Here's how the part is built. I have some questions about the finished solid (model axes, mm). Face numbers are marked on the shaded views. A direction names the side the tool comes from. Coordinates: 2 decimals unless noted, no trailing zeros. Write each loop counter-clockwise with the first axis right and the second up, starting at its lowest first coordinate (ties: lowest second). Pieces come first, ordered by that corner, then holes. Notation, with made-up numbers: (29, -1) -> (45, -1) arc R19 cw to (45, 16) -> close; hole circle Ø6 at (82.25, 82). An arc over 180 degrees is marked (long way). Use a Markdown table: item, result. Add a question column.
```python
from build123d import *

# Parameters (mm, degrees)
SKETCH1_W                  = 36.2966
SKETCH1_H                  = 80.2132
BOSS_BASE_DEPTH            = 2.1717
SKETCH3_W                  = 36.2966
SKETCH3_H                  = 2.1717
BOSS_LIP_DEPTH             = 23.25116
F_4_0_209_DIAMETER_HOLE1_D = 5.3086
F_4_0_209_DIAMETER_HOLE2_D = 5.3086
SKETCH19_W                 = 3.0734
SKETCH19_H                 = 66.04
CUT_EXTRUDE1_DEPTH         = 50.784702448
FILLET1_R                  = 3.81
FILLET4_R                  = 0.635


with BuildPart() as part:
    # Sketch1 → Boss-Base (new body)
    with BuildSketch(Plane(origin=(0, 0, 0), x_dir=(1, 0, 0), z_dir=(0, 1, 0))):
        Rectangle(SKETCH1_W, SKETCH1_H)
    extrude(amount=BOSS_BASE_DEPTH)

    # Sketch3 → Boss-Lip (add)
    with BuildSketch(Plane(origin=(0, 2.1717, 0), x_dir=(1, 0, 0), z_dir=(0, 1, 0))):
        with Locations((0, 39.02075)):
            Rectangle(SKETCH3_W, SKETCH3_H)
    extrude(amount=BOSS_LIP_DEPTH)

    # #4 (0.209) Diameter Hole1 (through all)
    with Locations(Plane(origin=(0, 2.1717, 0), x_dir=(1, 0, 0), z_dir=(0, 1, 0))):
        with Locations((0, -29.9466), (0, 10.0584)):
            Hole(F_4_0_209_DIAMETER_HOLE1_D / 2)

    # #4 (0.209) Diameter Hole2 (through all)
    with Locations(Plane.XY.offset(-37.9349)):
        with Locations((10.2743, 17.54886), (-10.2743, 17.54886)):
            Hole(F_4_0_209_DIAMETER_HOLE2_D / 2)

    # Sketch19 → Cut-Extrude1 (cut, through all)
    with BuildSketch(Plane(origin=(0, 2.1717, 0), x_dir=(1, 0, 0), z_dir=(0, 1, 0))):
        with Locations((16.6116, -7.0866)):
            Rectangle(SKETCH19_W, SKETCH19_H)
        with Locations((-16.6116, -7.0866)):
            Rectangle(SKETCH19_W, SKETCH19_H)
    extrude(amount=-CUT_EXTRUDE1_DEPTH, mode=Mode.SUBTRACT)

    # Fillet1
    # the kernel refuses this fillet: 3.81 mm, written as the material it adds along each edge
    with BuildSketch(Plane(origin=(18.1483, 2.1717, -37.9349), x_dir=(0, 0, 1), z_dir=(-1, 0, 0))) as fillet1_piece_1:
        with BuildLine():
            CenterArc((FILLET1_R, FILLET1_R), FILLET1_R, 180, 90)
            Line((0, FILLET1_R), (0, 0))
            Line((0, 0), (FILLET1_R, 0))
        make_face()
    extrude(amount=36.2966)
    # the kernel refuses this fillet: 3.81 mm, written as the material it takes off along each edge
    with BuildSketch(Plane(origin=(-18.1483, 11.51699308, -25.9334), x_dir=(0, 0, -1), z_dir=(0, -1, 0))) as fillet1_2_piece_1:
        with BuildLine():
            CenterArc((3.738117232, 3.81), FILLET1_R, 191.147377986, 78.852622014)
            Line((0, 3.0734), (0, 0))
            Line((0, 0), (3.738117232, 0))
        make_face()
    extrude(amount=20.86228616, mode=Mode.SUBTRACT)
    with BuildSketch(Plane(origin=(18.1483, 11.51699308, -25.9334), x_dir=(-1, 0, 0), z_dir=(0, -1, 0))) as fillet1_2_piece_2:
        with BuildLine():
            CenterArc((3.81, 3.738117232), FILLET1_R, 180, 78.852622014)
            Line((0, 3.738117232), (0, 0))
            Line((0, 0), (3.0734, 0))
        make_face()
    extrude(amount=20.86228616, mode=Mode.SUBTRACT)
    with BuildSketch(Plane(origin=(15.0749, 11.6967, 40.1066), x_dir=(-1, 0, 0), z_dir=(0, -1, 0))) as fillet1_2_piece_3:
        with BuildLine():
            CenterArc((FILLET1_R, FILLET1_R), FILLET1_R, 180, 90)
            Line((0, FILLET1_R), (0, 0))
            Line((0, 0), (FILLET1_R, 0))
        make_face()
    extrude(amount=21.2217, mode=Mode.SUBTRACT)
    with BuildSketch(Plane(origin=(-15.0749, 11.6967, 40.1066), x_dir=(1, 0, 0), z_dir=(0, -1, 0)), Plane(origin=(-18.1483, 25.42286, -28.4099), x_dir=(0, -1, 0), z_dir=(0, 0, -1)), Plane(origin=(18.1483, 25.42286, -49.6316), x_dir=(0, -1, 0), z_dir=(0, 0, 1))) as fillet1_2_piece_4:
        with BuildLine():
            CenterArc((FILLET1_R, -FILLET1_R), FILLET1_R, 90, 90)
            Line((0, -FILLET1_R), (0, 0))
            Line((0, 0), (FILLET1_R, 0))
        make_face()
    extrude(amount=21.2217, mode=Mode.SUBTRACT)
    with BuildSketch(Plane(origin=(-27.6733, 0, -40.1066), x_dir=(0, 0, 1), z_dir=(1, 0, 0))) as fillet1_2_piece_5:
        with BuildLine():
            CenterArc((FILLET1_R, -FILLET1_R), FILLET1_R, 90, 90)
            Line((0, -FILLET1_R), (0, 0))
            Line((0, 0), (FILLET1_R, 0))
        make_face()
    extrude(amount=55.3466, mode=Mode.SUBTRACT)

    # Fillet4
    fillet4_edges = [part.edges().sort_by_distance(p)[0] for p in [
        (18.1483, 3.287623164, -36.818976836),
        (-18.1483, 3.287623164, -36.818976836),
        (15.0749, 0, 5.1816),
        (15.0749, 2.1717, 5.1816),
        (18.1483, 13.79728, -37.9349),
        (0, 25.42286, -37.9349),
        (-18.1483, 13.79728, -37.9349),
        (17.032376836, 24.306936836, -37.9349),
        (-17.032376836, 24.306936836, -37.9349),
        (18.1483, 2.1717, -31.898208616),
        (-18.1483, 2.1717, -31.898208616),
        (-15.0749, 2.1717, 5.1816),
        (0, 2.1717, 40.1066),
        (-17.281304077, 2.1717, -27.251842254),
        (17.281304077, 2.1717, -27.251842254),
        (13.958976836, 2.1717, 38.990676836),
        (-13.958976836, 2.1717, 38.990676836),
        (-18.1483, 12.71143, -40.1066),
        (0, 25.42286, -40.1066),
        (18.1483, 12.71143, -40.1066),
        (17.032376836, 24.306936836, -40.1066),
        (-17.032376836, 24.306936836, -40.1066),
        (-18.1483, 0, -32.984058616),
        (-18.1483, 1.115923164, -38.990676836),
        (0, 0, 40.1066),
        (-15.0749, 0, 5.1816),
        (18.1483, 0, -32.984058616),
        (-17.281304077, 0, -27.251842254),
        (17.281304077, 0, -27.251842254),
        (13.958976836, 0, 38.990676836),
        (-13.958976836, 0, 38.990676836),
        (18.1483, 1.115923164, -38.990676836),
    ]]
    fillet(fillet4_edges, radius=FILLET4_R)


solid = part.part
```
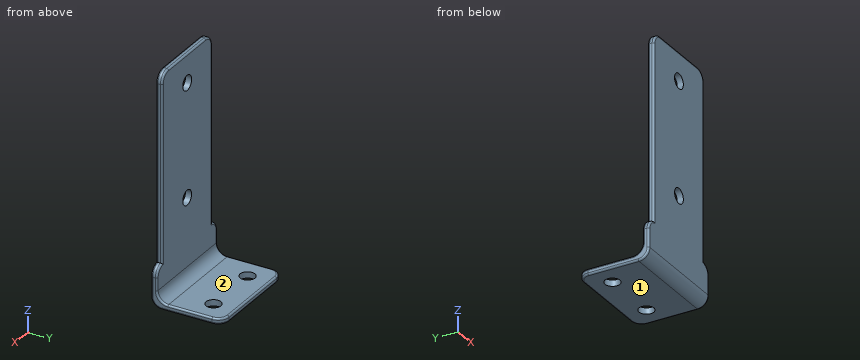
Q1. Which directions (+Z, -Z, +X, -X, +Y, -Y) give clear straight access to the entire face, cutting with the end or side of a thin tool? Please do the marked faces 1 and 2.
Q2. Suppose I cut it at D-D, the plane x = 5. Write out the boundary of the cut face in (y, z) (3 decimals).
Q3. Suppose I cut it at A-A, the plane x = 0. Write out the boundary of the cut face in (y, z) (3 decimals).
Q4. Suppose I cut it at B-B, the plane y = 16.5. Write out the boundary of the cut face in (x, z) (3 decimals).
Q5. Suppose I cut it at C-C, the plane z = 24. Write out the boundary of the cut face in (x, y) (3 decimals), and give its area (3 significant figures).
Q6. Please list where these lines run through material, in increasing order: line 1 (Z direction, x = 0, y = 1.45); line 2 (Y direction, x = 0, z = 8.5); line 3 (Z direction, x = 0, y = 1.25).
Q7. Will these pins go through, and if not, where does the flat tip stop? pin 1 (4 mm diameter, centred on x = 10.27, y = 17.55, fed in from -Z); pin 2 (3 mm diameter, centred on x = 9.5, z = -1.5, fed in from +Y); pin 3 (0.7 mm diameter, centred on y = 1, z = 10.5, fed in from +X); pin 4 (2 mm diameter, centred on x = -8, y = 19, fed in from +Z).
Answer key:
| question | item | result |
|---|---|---|
| 1 | face 1 | -Z, +X, -X, +Y, -Y |
| 1 | face 2 | +Z, +X, -X, +Y |
| 2 | outline | (0, -36.297) arc R3.81 ccw to (3.81, -40.107) -> (24.788, -40.107) arc R0.635 ccw to (25.423, -39.472) -> (25.423, -38.57) arc R0.635 ccw to (24.788, -37.935) -> (5.982, -37.935) arc R3.81 cw to (2.172, -34.125) -> (2.172, 39.472) arc R0.635 ccw to (1.537, 40.107) -> (0.635, 40.107) arc R0.635 ccw to (0, 39.472) -> close |
| 3 | outline | (0, -36.297) arc R3.81 ccw to (3.81, -40.107) -> (24.788, -40.107) arc R0.635 ccw to (25.423, -39.472) -> (25.423, -38.57) arc R0.635 ccw to (24.788, -37.935) -> (5.982, -37.935) arc R3.81 cw to (2.172, -34.125) -> (2.172, -12.713) -> (0, -12.713) -> close; (0, -7.404) -> (2.172, -7.404) -> (2.172, 27.292) -> (0, 27.292) -> close; (0, 32.601) -> (2.172, 32.601) -> (2.172, 39.472) arc R0.635 ccw to (1.537, 40.107) -> (0.635, 40.107) arc R0.635 ccw to (0, 39.472) -> close |
| 4 | outline | (-18.148, -39.472) arc R0.635 ccw to (-17.513, -40.107) -> (-12.713, -40.107) -> (-12.713, -37.935) -> (-17.513, -37.935) arc R0.635 ccw to (-18.148, -38.57) -> close; (-7.836, -40.107) -> (7.836, -40.107) -> (7.836, -37.935) -> (-7.836, -37.935) -> close; (12.713, -40.107) -> (17.513, -40.107) arc R0.635 ccw to (18.148, -39.472) -> (18.148, -38.57) arc R0.635 ccw to (17.513, -37.935) -> (12.713, -37.935) -> close |
| 5 | outline | (-15.075, 0.635) arc R0.635 ccw to (-14.44, 0) -> (14.44, 0) arc R0.635 ccw to (15.075, 0.635) -> (15.075, 1.537) arc R0.635 ccw to (14.44, 2.172) -> (-14.44, 2.172) arc R0.635 ccw to (-15.075, 1.537) -> close |
| 5 | area | 65.1 mm^2 |
| 6 | line 1 | z = -39.29 to -12.71, -7.4 to 27.29, 32.6 to 40.11 |
| 6 | line 2 | y = 0 to 2.17 |
| 6 | line 3 | z = -39.12 to -12.71, -7.4 to 27.29, 32.6 to 40.11 |
| 7 | pin 1 | passes through |
| 7 | pin 2 | stops at y = 2.17 |
| 7 | pin 3 | stops at x = 15.07 |
| 7 | pin 4 | stops at z = -37.93 |
